```python
from build123d import *

# Parameters (mm, degrees)
F0_R     = 25.1419011997
F1_DEPTH = 127
F4_R     = 5.08
F5_SIZE  = 5.08


with BuildPart() as f1:
    # F0 (on Top) → F1 (new body)
    with BuildSketch(Plane.XY):
        Circle(F0_R)
    extrude(amount=F1_DEPTH)

    # F0 (on Top) → F3 section 0
    with BuildSketch(Plane.XY, mode=Mode.PRIVATE) as f3_s0:
        Circle(F0_R)
    loft([f3_s0.sketch, Vertex(0, 0, -37.6585572958)])

    # F4
    f4_edges = [f1.edges().sort_by_distance(p)[0] for p in [
        (-25.141901, 0, 0),
    ]]
    fillet(f4_edges, radius=F4_R)

    # F5
    f5_edges = [f1.edges().sort_by_distance(p)[0] for p in [
        (-25.141901, 0, 127),
    ]]
    chamfer(f5_edges, length=F5_SIZE)


solid = f1.part
```
The model under review builds one solid part; all positions refer to its coordinate system, in mm. Round coordinates to 2 decimals unless told otherwise and drop trailing zeros. Order: outer loops, then holes, each group sorted by start corner. A loop starts at its lowest first (then second) coordinate and runs counter-clockwise, first axis right, second up. Notation, with made-up numbers: (-24.75, 56) - (-13.75, 56) arc R18 ccw to (-13.75, 71) - close; hole circle Ø10 at (13.25, -14). An arc over 180 degrees is marked (long way). Answer in a Markdown table with one row per item.
(1) Take a section at A-A on z = 4. Write out the cut boundary in (x, y).
Result set:
| item | result |
|---|---|
| outline | circle Ø50.28 at (0, 0) |
(2) For line 1 (Y direction, x = 1, z = 102.5); line 2 (X direction, y = -6.5, z = 85.5); line 3 (Y direction, x = -17, z = 15.5), list the stretches that pass through material, from the lowest coordinate up. Write a range as from..to.
Result set:
| item | result |
|---|---|
| line 1 | y = -25.12..25.12 |
| line 2 | x = -24.29..24.29 |
| line 3 | y = -18.52..18.52 |
(3) Take a section at B-B on z = -19. Write out the cut boundary in (x, y), plus the area to 4 significant figures.
Result set:
| item | result |
|---|---|
| outline | circle Ø24.91 at (0, 0) |
| area | 487.5 mm2 |
(4) Clearance check with flat-ended pins moving along their axes: P1, Ø8, axis at y = -18, z = 8, coming from the +X side; P2, Ø3, axis at y = -12, z = 78, coming from the -X side; P3, Ø12, axis at x = 15, z = -7, coming from the +Y side. State where each tip first meets the part, or that it passes through.
Result set:
| item | result |
|---|---|
| P1 | stops at x = 20.88 |
| P2 | stops at x = -22.84 |
| P3 | stops at y = 20.75 |
